Geometry check sheet. Reference: the model listing, model coordinates, mm. A direction names the side the tool comes from. Give positions to 0.01 mm unless a question says otherwise; leave off trailing zeros. Write each loop counter-clockwise with the first axis right and the second up, starting at its lowest first coordinate (ties: lowest second). Pieces come first, ordered by that corner, then holes. Notation, with made-up numbers: (72.5, -5.5) - (108.5, -5.5) arc R20 ccw to (108.5, 14.5) - close; hole circle Ø5 at (73.25, 68). An arc over 180 degrees is marked (long way). Use a Markdown table: item, result.
```python
from build123d import *

# Parameters (mm, degrees)
F0_R     = 2.75
F0_R_2   = 1.5
F1_DEPTH = 9
F0_R_3   = 3.5
F2_DEPTH = 1
F0_R_4   = 4.9
F3_DEPTH = 20
F4_SIZE  = 1
F5_SIZE  = 0.6
F6_SIZE  = 0.4


with BuildPart() as f1:
    # F0 (on Top) → F1 (new body)
    with BuildSketch(Plane.XY):
        Circle(F0_R)
        Circle(F0_R_2, mode=Mode.SUBTRACT)
    extrude(amount=-F1_DEPTH)

    # F0 (on Top) → F2 (join)
    with BuildSketch(Plane.XY):
        Circle(F0_R_3)
        Circle(F0_R, mode=Mode.SUBTRACT)
        Circle(F0_R)
        Circle(F0_R_2, mode=Mode.SUBTRACT)
    extrude(amount=F2_DEPTH)

    # F0 (on Top) → F3 (join)
    with BuildSketch(Plane.XY):
        Circle(F0_R_4)
        Circle(F0_R_3, mode=Mode.SUBTRACT)
    extrude(amount=F3_DEPTH)

    # F4
    f4_edges = [f1.edges().sort_by_distance(p)[0] for p in [
        (-4.9, 0, 0),
    ]]
    chamfer(f4_edges, length=F4_SIZE)

    # F5
    f5_edges = [f1.edges().sort_by_distance(p)[0] for p in [
        (-1.5, 0, 1),
    ]]
    chamfer(f5_edges, length=F5_SIZE)

    # F6
    f6_edges = [f1.edges().sort_by_distance(p)[0] for p in [
        (-2.75, 0, -9),
    ]]
    chamfer(f6_edges, length=F6_SIZE)


solid = f1.part
```
1) Material ranges on L1, parallel to Y at x = 0, z = 16; L2, parallel to Y at x = 0, z = -3.5; L3, parallel to X at y = -0.5, z = 17.75, recorded low to high. Write a range as from..to.
Working result:
| item | result |
|---|---|
| L1 | y = -4.9..-3.5, 3.5..4.9 |
| L2 | y = -2.75..-1.5, 1.5..2.75 |
| L3 | x = -4.87..-3.46, 3.46..4.87 |
2) Mould release check, pull along X, two halves, no side actions. Record for faces 3 (the flat face through (1, 3, 0)), 4 (the cylindrical face through (3.233, -1.341, 10.367)), 5 (the cylindrical face through (-0.596, -2.685, -4.24)): pulls with the +X half, pulls with the -X half, needs draft (parallel to the pull), parting line crosses it, or undercut.
Working result:
| item | result |
|---|---|
| face 3 | needs draft |
| face 4 | undercut |
| face 5 | parting line crosses it |
3) Set-up check for faces 1 (the flat face through (2, -2, 1)), 2 (the cylindrical face through (-1.5, 0.07, -4.37)): record each of +Z, -Z, +X, -X, +Y, -Y from which the full face is reachable in a straight line by a thin tool's end or side.
Working result:
| item | result |
|---|---|
| face 1 | +Z |
| face 2 | +Z, -Z |
4) Section check A-A on y = 0. Record the boundary of the cut face in (x, z).
Working result:
| item | result |
|---|---|
| outline | (-4.9, 1) - (-3.9, 0) - (-2.75, 0) - (-2.75, -8.6) - (-2.35, -9) - (-1.5, -9) - (-1.5, 0.4) - (-2.1, 1) - (-3.5, 1) - (-3.5, 20) - (-4.9, 20) - close; (1.5, -9) - (2.35, -9) - (2.75, -8.6) - (2.75, 0) - (3.9, 0) - (4.9, 1) - (4.9, 20) - (3.5, 20) - (3.5, 1) - (2.1, 1) - (1.5, 0.4) - close |
5) Depth check by flat-ended pin: P1, Ø1, axis at x = -1.5, z = 2.5, coming from the -Y side; P2, Ø2, axis at x = -1, y = -1, coming from the +Z side. Enter the tip coordinate at first touch or a pass-through.
Working result:
| item | result |
|---|---|
| P1 | stops at y = -4.8 |
| P2 | stops at z = 1 |
6) Section check D-D on z = 12.25. Record the boundary of the cut face in (x, y), then the cut area to 3 significant figures.
Working result:
| item | result |
|---|---|
| outline | circle Ø9.8 at (0, 0); hole circle Ø7 at (0, 0) |
| area | 36.9 mm² |
7) Section check C-C on z = -3.25. Record the boundary of the cut face in (x, y).
Working result:
| item | result |
|---|---|
| outline | circle Ø5.5 at (0, 0); hole circle Ø3 at (0, 0) |
